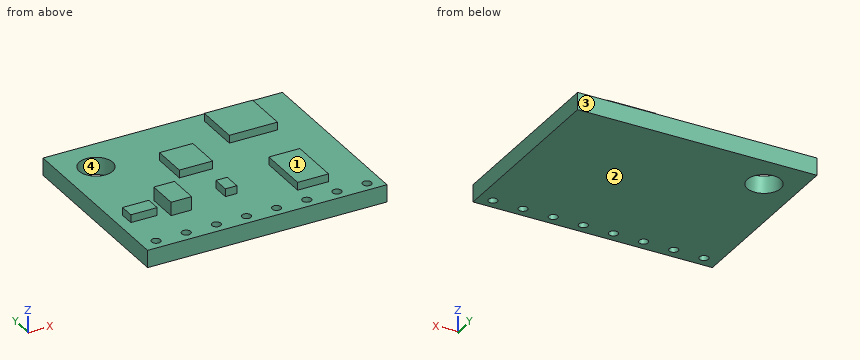
from build123d import *

# Parameters (mm, degrees)
F0_W     = 21.43
F0_H     = 16.8
F0_R     = 0.4
F0_R_2   = 1.5
F1_DEPTH = 0.775
F2_W     = 2.359656
F2_H     = 1.333718
F2_W_2   = 1.025936
F2_H_2   = 1.538906
F2_W_3   = 2.975217
F2_H_3   = 3.180405
F2_W_4   = 2.770032
F2_H_4   = 4.616717
F2_W_5   = 4.308936
F2_H_5   = 4.001155
F3_DEPTH = 0.7
F2_W_6   = 1.846687
F2_H_6   = 2.770031
F4_DEPTH = 1.2


with BuildPart() as f1:
    # F0 (on Top) → F1 (new body, symmetric)
    with BuildSketch(Plane.XY):
        Rectangle(F0_W, F0_H)
        with Locations((-9.393446, -7.391692)):
            Circle(F0_R, mode=Mode.SUBTRACT)
        with Locations((-6.7, -7.4)):
            Circle(F0_R, mode=Mode.SUBTRACT)
        with Locations((-4.006554, -7.408308)):
            Circle(F0_R, mode=Mode.SUBTRACT)
        with Locations((-1.313108, -7.416616)):
            Circle(F0_R, mode=Mode.SUBTRACT)
        with Locations((1.380338, -7.424924)):
            Circle(F0_R, mode=Mode.SUBTRACT)
        with Locations((4.073785, -7.433231)):
            Circle(F0_R, mode=Mode.SUBTRACT)
        with Locations((6.767231, -7.441539)):
            Circle(F0_R, mode=Mode.SUBTRACT)
        with Locations((9.460677, -7.449847)):
            Circle(F0_R, mode=Mode.SUBTRACT)
        with Locations((-7.768597, 5.178844)):
            Circle(F0_R_2, mode=Mode.SUBTRACT)
    extrude(amount=F1_DEPTH, both=True)

    # F2 (on face) → F3 (join)
    with BuildSketch(Plane.XY.offset(0.775)):
        with Locations((-8.531306, -3.239972)):
            Rectangle(F2_W, F2_H)
        with Locations((-0.734184, -3.137378)):
            Rectangle(F2_W_2, F2_H_2)
        with Locations((-1.452339, 2.043604)):
            Rectangle(F2_W_3, F2_H_3)
        with Locations((5.57533, -3.445159)):
            Rectangle(F2_W_4, F2_H_4)
        with Locations((5.318846, 5.3779)):
            Rectangle(F2_W_5, F2_H_5)
    extrude(amount=F3_DEPTH)

    # F2 (on face) → F4 (join)
    with BuildSketch(Plane.XY.offset(0.775)):
        with Locations((-5.504791, -3.086081)):
            Rectangle(F2_W_6, F2_H_6)
    extrude(amount=F4_DEPTH)


solid = f1.part
The listing builds one solid part. Answer for the finished solid, in the listing's coordinates (mm). Face numbers are marked on the shaded views. A direction names the side the tool comes from. Give positions to 0.01 mm unless a question says otherwise; leave off trailing zeros. Write each loop counter-clockwise with the first axis right and the second up, starting at its lowest first coordinate (ties: lowest second). Pieces come first, ordered by that corner, then holes. Notation, with made-up numbers: (62.5, -18.75) - (67.5, -18.75) arc R6 cw to (67.5, -11.75) - close; hole circle Ø1 at (29.5, 65). An arc over 180 degrees is marked (long way). One line per question, with ' | ' between items. Start each with the question number.
1. Section D-D, the plane z = -0.25 is taken. Count the separate pieces of the cut face and the enclosed holes in it, then the cut area to 3 significant figures.
2. Section A-A, the plane y = 5.5 is taken. Determine the outline of the cut face in (x, z) (3 decimals), then the cut area to 3 significant figures.
3. Determine the mould class of the marked faces 3 and 4 for opening direction X: +X half, -X half, draft (parallel to the pull), parting line (faces both ways), or undercut.
4. For the marked faces 1 and 2, determine the directions among +Z, -Z, +X, -X, +Y, -Y from which every point of the face is accessible in a straight line to the end or side of a thin tool.
5. Section C-C, the plane x = -6.7 is taken. Determine the outline of the cut face in (y, z) (1 decimal), then the cut area to 3 significant figures.
6. Section B-B, the plane y = -5.5 is taken. Determine the outline of the cut face in (x, z) (3 decimals).
7. Straight lines are drawn through the part: line 1 (X direction, y = -3.25, z = 1.35); line 2 (Y direction, x = -7, z = -0.45); line 3 (Z direction, x = 7.5, y = -3.75) (3 decimals). For each, find the intervals that lie inside material, in ascending order.
8. Given P1, Ø1.3, axis at y = -3.5, z = 1.5, coming from the -X side; P2, Ø0.9, axis at x = -1, y = 1.5, coming from the +Z side (3 decimals); P3, Ø2, axis at x = 1, y = -3.5, coming from the +Z side (3 decimals), each flat-ended and moving along its own axis, determine where each tip first touches the part or whether it passes through.
Result:
1) separate pieces: 1 | enclosed holes: 9 | area: 349 mm2
2) outline: (-10.715, -0.775) - (-9.234, -0.775) - (-9.234, 0.775) - (-10.715, 0.775) - close; (-6.303, -0.775) - (10.715, -0.775) - (10.715, 0.775) - (7.473, 0.775) - (7.473, 1.475) - (3.164, 1.475) - (3.164, 0.775) - (-6.303, 0.775) - close | area: 31.7 mm2
3) face 3: draft | face 4: undercut
4) face 1: +Z, +X, +Y, -Y | face 2: -Z, +X, -X, +Y, -Y
5) outline: (-8.4, -0.8) - (-7.8, -0.8) - (-7.8, 0.8) - (-8.4, 0.8) - close; (-7, -0.8) - (4.1, -0.8) - (4.1, 0.8) - (-7, 0.8) - close; (6.2, -0.8) - (8.4, -0.8) - (8.4, 0.8) - (6.2, 0.8) - close | area: 21.5 mm2
6) outline: (-10.715, -0.775) - (10.715, -0.775) - (10.715, 0.775) - (6.96, 0.775) - (6.96, 1.475) - (4.19, 1.475) - (4.19, 0.775) - (-10.715, 0.775) - close
7) line 1: x = -9.71 to -7.35, -6.43 to -4.58, -1.25 to -0.22, 4.19 to 6.96 | line 2: y = -8.4 to -7.66, -7.14 to 3.89, 6.47 to 8.4 | line 3: z = -0.775 to 0.775
8) P1: stops at x = -9.71 | P2: stops at z = 1.475 | P3: stops at z = 0.775
